Design review of the part built by this model. Coordinates are the model's own, in mm. A direction names the side the tool comes from. Coordinates: 2 decimals unless noted, no trailing zeros. Write each loop counter-clockwise with the first axis right and the second up, starting at its lowest first coordinate (ties: lowest second). Pieces come first, ordered by that corner, then holes. Notation, with made-up numbers: (29, 62.5) - (40, 62.5) arc R22 ccw to (40, 92.5) - close; hole circle Ø2 at (36.25, 13). An arc over 180 degrees is marked (long way). Use a Markdown table: item, result.
from build123d import *

# Parameters (mm, degrees)
F0_R        = 12.5
F1_DEPTH    = 15
F2_R        = 5.35
F3_DEPTH    = 19.7
F4_R        = 11.5
F5_DEPTH    = 2
F6_T1_DEPTH = 43.3845163924
F6_T3_DEPTH = 43.3709168199
F8_DEPTH    = 41


# Not quite as in the source:
# - a fillet or chamfer that OpenCascade refuses, or shapes differently, is made with other operations: its cross-section is extruded or revolved along the edge and cut away or added


with BuildPart() as f1:
    # F0 (on Top) → F1 (new body)
    with BuildSketch(Plane.XY):
        Circle(F0_R)
    extrude(amount=F1_DEPTH)

    # F2 (on Front) → F3 (cut, symmetric)
    with BuildSketch(Plane.XZ):
        with Locations((0.0221527088, 9.997321542)):
            Circle(F2_R)
    extrude(amount=F3_DEPTH, both=True, mode=Mode.SUBTRACT)

    # F4 (on Top) → F5 (cut)
    with BuildSketch(Plane.XY):
        Circle(F4_R)
    extrude(amount=F5_DEPTH, mode=Mode.SUBTRACT)

    # F6: chamfer of 7 on 2 edges, made by hand

    # F6_s2 → F6_t1 (cut)
    with BuildSketch(Plane.XZ.offset(-21.6922581962)):
        with BuildLine():
            Line((-4.2755328164, 12.7512221633), (-5.5992962087, 15.2473673359))
            Line((-5.5992962087, 15.2473673359), (-5.5992962087, 15.3873673359))
            ThreePointArc((-5.5992962087, 15.3873673359), (-3.7366893911, 15.14), (-1.8740825735, 15.14))
            Line((-1.8740825735, 15.14), (-1.8244614633, 14.869088788))
            ThreePointArc((-1.8244614633, 14.869088788), (-3.2288770936, 14.0685504994), (-4.1596371494, 12.6726843102))
            Line((-4.1596371494, 12.6726843102), (-4.2755328164, 12.7512221633))
        make_face()
    extrude(amount=F6_T1_DEPTH, mode=Mode.SUBTRACT)

    # F6_s4 → F6_t3 (cut)
    with BuildSketch(Plane.XZ.offset(-21.6854584099)):
        with BuildLine():
            Line((5.6436016264, 15.2473673359), (4.3198382341, 12.7512221633))
            Line((4.3198382341, 12.7512221633), (4.2039425671, 12.6726843102))
            ThreePointArc((4.2039425671, 12.6726843102), (3.2731825113, 14.0685504994), (1.868766881, 14.869088788))
            Line((1.868766881, 14.869088788), (1.9183879912, 15.14))
            ThreePointArc((1.9183879912, 15.14), (3.7809948088, 15.14), (5.6436016264, 15.3873673359))
            Line((5.6436016264, 15.3873673359), (5.6436016264, 15.2473673359))
        make_face()
    extrude(amount=F6_T3_DEPTH, mode=Mode.SUBTRACT)

    # F7 (on Front) → F8 (cut, symmetric)
    with BuildSketch(Plane.XZ):
        Polygon((22.090458405, 20.6357296556), (7.1151317097, 20.4473696649), (14.5756583661, -3.0394739006), align=None)
        Polygon((-14.5756583661, -3.0394739006), (-7.1151317097, 20.4473696649), (-22.090458405, 20.6357296556), align=None)
    extrude(amount=F8_DEPTH, both=True, mode=Mode.SUBTRACT)


solid = f1.part
(1) Take a section at C-C on x = -1.75. Write out the cut boundary in (y, z).
Determined:
| item | result |
|---|---|
| outline | (-12.38, 0) - (-11.37, 0) - (-11.37, 2) - (11.37, 2) - (11.37, 0) - (12.38, 0) - (12.38, 4.95) - (-12.38, 4.95) - close |
(2) Draft analysis for pull direction X (two halves, no side actions). For faces 1 (the flat face through (0, 0, 2)), 2 (the flat face through (11, -4, 0)), 3 (the cylindrical face through (11.547, -4.788, 5.728)), state which applies: +X half, -X half, draft (parallel to the pull), parting line (faces both ways), or undercut.
Determined:
| item | result |
|---|---|
| face 1 | undercut |
| face 2 | draft |
| face 3 | parting line |
(3) Take a section at D-D on z = 10. Write out the cut boundary in (x, y), and give its area (3 significant figures).
Determined:
| item | result |
|---|---|
| outline | (-10.43, -6.88) arc R12.5 ccw to (-5.33, -11.31) - (-5.33, 11.31) arc R12.5 ccw to (-10.43, 6.88) - close; (5.37, -11.29) arc R12.5 ccw to (10.43, -6.88) - (10.43, 6.88) arc R12.5 ccw to (5.37, 11.29) - close |
| area | 193 mm2 |
(4) Take a section at B-B on z = 8. Write out the cut boundary in (x, y).
Determined:
| item | result |
|---|---|
| outline | (-11.07, -5.81) arc R12.5 ccw to (-4.94, -11.48) - (-4.94, 11.48) arc R12.5 ccw to (-11.07, 5.81) - close; (4.99, -11.46) arc R12.5 ccw to (11.07, -5.81) - (11.07, 5.81) arc R12.5 ccw to (4.99, 11.46) - close |
(5) For L1, parallel to Y at x = 0, z = 0.9; L2, parallel to X at y = -10.5, z = 1.25; L3, parallel to X at y = 5, z = 11.5, list the stretches that pass through material, from the lowest coordinate up. Write a range as from..to.
Determined:
| item | result |
|---|---|
| L1 | -12.5..-11.5, 11.5..12.5 |
| L2 | -6.78..-4.69, 4.69..6.78 |
| L3 | -9.96..-5.11, 5.16..9.96 |
(6) Take a section at A-A on y = 0. Write out the cut boundary in (x, z) (3 decimals).
Determined:
| item | result |
|---|---|
| outline | (-12.5, 0) - (-11.5, 0) - (-11.5, 2) - (11.5, 2) - (11.5, 0) - (12.5, 0) - (12.5, 3.495) - (8.845, 15) - (5.512, 15) - (4.451, 12.999) arc R5.35 cw (long way) to (-4.407, 12.999) - (-5.468, 15) - (-8.845, 15) - (-12.5, 3.495) - close |
(7) For pin 1 (1.5 mm diameter, centred on x = -0.5, y = 5, fed in from +Z); pin 2 (6 mm diameter, centred on y = 7, z = 10, fed in from +X); pin 3 (4 mm diameter, centred on x = 7, z = 7, fed in from +Y), all flat-tipped, find the tip position at first contact; note any pin that passes through.
Determined:
| item | result |
|---|---|
| pin 1 | z = 4.8 |
| pin 2 | x = 11.25 |
| pin 3 | y = 11.46 |
(8) Machinability: for faces 4 (the flat face through (7, 0, 15)), 5 (the flat face through (4.989, 0.164, 14.013)), 6 (the cylindrical face through (-1.5, 11.4, 1)), which of the approach directions +Z, -Z, +X, -X, +Y, -Y give a long, thin tool a straight path to every point of the face, cutting with its end or side? Answer none if there is none.
Determined:
| item | result |
|---|---|
| face 4 | +Z, +X, -X, +Y, -Y |
| face 5 | +Z, +Y, -Y |
| face 6 | -Z |
